```python
from build123d import *

# Parameters (mm, degrees)
SKETCH2_W                       = 27.178
SKETCH2_H                       = 21.59
INITIAL_EXTRUDE_DEPTH           = 6.35
SKETCH3_W                       = 27.178
SKETCH3_H                       = 1.27
INTIAL_EXTRUDE_HORIZONTAL_DEPTH = 12.192
SKETCH4_W                       = 27.178
SKETCH4_H                       = 1.27
SLIGHT_EXTRUDE_VERTICAL_DEPTH   = 0.254
SKETCH5_W                       = 3.048
SKETCH5_H                       = 21.59
CUT_EXTRUDE1_DEPTH              = 2.794
CUT_EXTRUDE2_REACH              = 33.537
SKETCH6_W                       = 1.379153921
SKETCH6_H                       = 12.954
SNAP_START                      = 11.473246079
SNAP_HOOK2_DEPTH                = 0.7366
SNAP_START_2                    = 8.31223189
SNAP_HOOK2_2_DEPTH              = 8.568362063
SNAP_START_3                    = 8.179116131
SNAP_HOOK2_3_DEPTH              = 8.834593581
SNAP_START_4                    = 9
SNAP_HOOK2_4_DEPTH              = 6
BOSS_EXTRUDE1_DEPTH             = 7.54
SKETCH8_W                       = 24.419692158
SKETCH8_H                       = 7.195933706
CUT_EXTRUDE3_DEPTH              = 0.762
SKETCH9_W                       = 24.419692158
SKETCH9_H                       = 20.32
BOSS_EXTRUDE2_DEPTH             = 2.794
SKETCH10_R                      = 5.08
CUT_EXTRUDE4_DEPTH              = 5.08


with BuildPart() as part:
    # Sketch2 → Initial Extrude (new body)
    with BuildSketch(Plane.XY):
        Rectangle(SKETCH2_W, SKETCH2_H)
    extrude(amount=INITIAL_EXTRUDE_DEPTH)

    # Sketch3 → Intial Extrude horizontal (add)
    with BuildSketch(Plane.XY.offset(6.35)):
        with Locations((0, 10.16)):
            Rectangle(SKETCH3_W, SKETCH3_H)
    extrude(amount=INTIAL_EXTRUDE_HORIZONTAL_DEPTH)

    # Sketch4 → Slight Extrude vertical (add)
    with BuildSketch(Plane.XZ.offset(-9.525)):
        with Locations((0, 17.907)):
            Rectangle(SKETCH4_W, SKETCH4_H)
    extrude(amount=SLIGHT_EXTRUDE_VERTICAL_DEPTH)

    # Sketch5 → Cut-Extrude1 (cut)
    with BuildSketch(Plane.ZY.offset(13.589)):
        with Locations((4.064, 0)):
            Rectangle(SKETCH5_W, SKETCH5_H)
    cut_extrude1 = extrude(amount=-CUT_EXTRUDE1_DEPTH, mode=Mode.SUBTRACT)

    # Mirror3: Cut-Extrude1 across plane
    add(cut_extrude1.mirror(Plane(origin=(0, 0, 0), x_dir=(0, 0, 1), z_dir=(1, 0, 0))), mode=Mode.SUBTRACT)

    # Sketch6 → Cut-Extrude2 (cut, up to next)
    with BuildSketch(Plane(origin=(0, 10.795, 0), x_dir=(1, 0, 0), z_dir=(0, 1, 0)), mode=Mode.PRIVATE) as cut_extrude2_sk1:
        with Locations((12.89942304, -12.065)):
            Rectangle(SKETCH6_W, SKETCH6_H)
    cut_extrude2_tool1 = extrude(cut_extrude2_sk1.sketch, amount=-CUT_EXTRUDE2_REACH, mode=Mode.PRIVATE) & part.part
    cut_extrude2 = cut_extrude2_tool1.solids().sort_by_distance((12.899423, 10.795, 12.065))[0]
    add(cut_extrude2, mode=Mode.SUBTRACT)

    # Mirror7: Cut-Extrude2 across plane
    add(cut_extrude2.mirror(Plane(origin=(0, 0, 0), x_dir=(0, 0, 1), z_dir=(1, 0, 0))), mode=Mode.SUBTRACT)

    # Snap Hook2: read off the stored shape, not the designer's step
    # Snap Hook2 outline → Snap Hook2 (add)
    with BuildSketch(Plane.YZ.offset(SNAP_START)):
        Polygon((10.795, 17.013709712), (10.795, 8.179116131), (15.113, 8.405412922), (15.113, 16.787412922), align=None)
    snap_hook2 = extrude(amount=SNAP_HOOK2_DEPTH)

    # Snap Hook2 2 outline → Snap Hook2 2 (add)
    with BuildSketch(Plane.XY.offset(SNAP_START_2)):
        Polygon((11.473246079, 10.795), (11.473246079, 15.113), (10.177846079, 10.795), align=None)
        Polygon((12.209846079, 15.113), (12.209846079, 13.335), (14.241846079, 13.335), (14.241846079, 14.605), align=None)
    snap_hook2_2 = extrude(amount=SNAP_HOOK2_2_DEPTH)

    # Snap Hook2 3 outline → Snap Hook2 3 (add)
    with BuildSketch(Plane.XY.offset(SNAP_START_3)):
        Polygon((11.473246079, 10.795), (11.473246079, 15.113), (10.177846079, 10.795), align=None)
    snap_hook2_3 = extrude(amount=SNAP_HOOK2_3_DEPTH)

    # Snap Hook2 4 outline → Snap Hook2 4 (cut)
    with BuildSketch(Plane.YZ.offset(SNAP_START_4)):
        Polygon((10.795, 8.179116131), (17, 8.179116131), (17, 8.504306402), (15.113, 8.405412922), align=None)
        Polygon((15.113, 16.787412922), (17, 16.688519443), (17, 17.013709712), (10.795, 17.013709712), align=None)
    snap_hook2_4 = extrude(amount=SNAP_HOOK2_4_DEPTH, mode=Mode.SUBTRACT)

    # Mirror6: Snap Hook2, Snap Hook2 2, Snap Hook2 3, Snap Hook2 4 across plane
    add(snap_hook2.mirror(Plane(origin=(0, 0, 0), x_dir=(0, 0, 1), z_dir=(1, 0, 0))))
    add(snap_hook2_2.mirror(Plane(origin=(0, 0, 0), x_dir=(0, 0, 1), z_dir=(1, 0, 0))))
    add(snap_hook2_3.mirror(Plane(origin=(0, 0, 0), x_dir=(0, 0, 1), z_dir=(1, 0, 0))))
    add(snap_hook2_4.mirror(Plane(origin=(0, 0, 0), x_dir=(0, 0, 1), z_dir=(1, 0, 0))), mode=Mode.SUBTRACT)

    # Sketch7 → Boss-Extrude1 (add)
    with BuildSketch(Plane(origin=(0, 10.795, 0), x_dir=(1, 0, 0), z_dir=(0, 1, 0))):
        Polygon((-8.962447439, -8.179116131), (-8.962447439, -18.542), (8.962447439, -18.542), (8.962447439, -8.179116131), (9, -8.179116131), (10.177846079, -8.179116131), (12.209846079, -8.179116131), (12.209846079, -5.588), (10.795, -5.588), (10.795, -2.54), (13.589, -2.54), (13.589, 0), (-13.589, 0), (-13.589, -2.54), (-10.795, -2.54), (-10.795, -5.588), (-12.209846079, -5.588), (-12.209846079, -8.179116131), (-10.177846079, -8.179116131), (-9, -8.179116131), align=None)
    extrude(amount=BOSS_EXTRUDE1_DEPTH)

    # Sketch8 → Cut-Extrude3 (cut)
    with BuildSketch(Plane.XZ.offset(-9.525)):
        with Locations((0, 13.674033147)):
            Rectangle(SKETCH8_W, SKETCH8_H)
    extrude(amount=-CUT_EXTRUDE3_DEPTH, mode=Mode.SUBTRACT)

    # Sketch9 → Boss-Extrude2 (add)
    with BuildSketch(Plane.XY.offset(6.35)):
        with Locations((0, -0.635)):
            Rectangle(SKETCH9_W, SKETCH9_H)
    extrude(amount=BOSS_EXTRUDE2_DEPTH)

    # Sketch10 → Cut-Extrude4 (cut)
    with BuildSketch(Plane(origin=(0, 18.335, 0), x_dir=(1, 0, 0), z_dir=(0, 1, 0))):
        with Locations(Location((0, -12.7, 0), (0, 0, 270))):
            Circle(SKETCH10_R)
    extrude(amount=-CUT_EXTRUDE4_DEPTH, mode=Mode.SUBTRACT)


solid = part.part
```
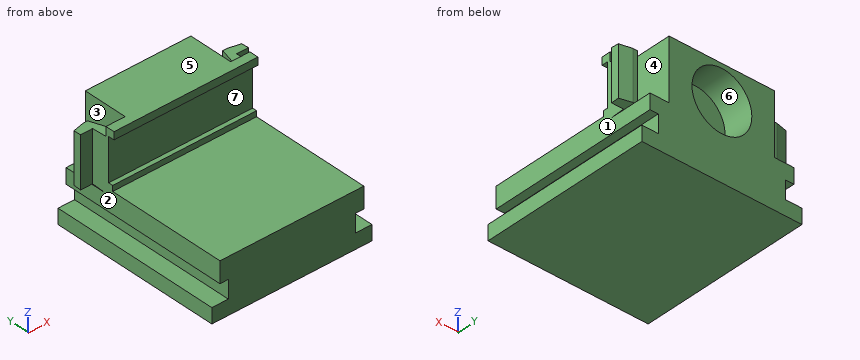
Could you check a few things on this model? Use its own coordinates, in mm. Face numbers are marked on the shaded views. A direction names the side the tool comes from. Coordinates: 2 decimals unless noted, no trailing zeros. Order: outer loops, then holes, each group sorted by start corner. A loop starts at its lowest first (then second) coordinate and runs counter-clockwise, first axis right, second up. Notation, with made-up numbers: M 52.5,-34.5 L 71.5,-34.5 A11 ccw 71.5,-24.5 Z; hole C -37,22 d2. An arc over 180 degrees is marked long. Use one line per item in the form item = value. Start each with the question number.
1. Please list where these lines run through material, in increasing order: line 1 (X direction, y = 16.5, z = 12.7); line 2 (Z direction, x = 9.75, y = 10); line 3 (X direction, y = 14.25, z = 15).
2. Suppose I cut it at C-C on y = -2.5. Write out the boundary of the cut face in (x, z) (3 decimals), then the cut area to 3 significant figures.
3. Suppose I cut it at D-D on z = 16. Write out the boundary of the cut face in (x, y) (3 decimals), then the cut area to 3 significant figures.
4. We'd pull the mould along X, two halves only. Please class the marked faces 1, 2, 3 and 4: +X half, -X half, draft (parallel to the pull), parting line (faces both ways), or undercut.
5. Suppose I cut it at A-A on x = 0. Write out the boundary of the cut face in (y, z) (3 decimals), then the cut area to 3 significant figures.
6. For pin 1 (3 mm diameter, centred on x = 11.5, y = 5.5, fed in from +Z); pin 2 (1 mm diameter, centred on x = 11, y = 15, fed in from +Z); pin 3 (1.5 mm diameter, centred on y = 11, z = 11, fed in from +X), each with a flat end and sliding along its axis, tell me the tip position at first contact or that it passes through.
7. On a 3-axis mill with a long thin cutter (end or side, diameter ignored), from which of +Z, -Z, +X, -X, +Y, -Y can I reach the whole of each face in a straight line? I mean the marked faces 5, 6 and 7. Say none if no direction works.
8. Suppose I cut it at B-B on z = 12.7. Write out the boundary of the cut face in (x, y) (3 decimals).
Geometry says:
q1.line_1 = -8.96 to -5.08, 5.08 to 8.96
q1.line_2 = 0 to 10.08, 17.27 to 18.54
q1.line_3 = -14.24 to -11.21, -8.96 to -4.53, 4.53 to 8.96, 11.21 to 14.24
q2.outline = M -13.589,0 L 13.589,0 L 13.589,2.54 L 10.795,2.54 L 10.795,5.588 L 12.21,5.588 L 12.21,9.144 L -12.21,9.144 L -12.21,5.588 L -10.795,5.588 L -10.795,2.54 L -13.589,2.54 Z
q2.area = 222 mm^2
q3.outline = M -14.242,13.335 L -12.21,13.335 L -12.21,10.287 L 12.21,10.287 L 12.21,13.335 L 14.242,13.335 L 14.242,14.605 L 12.21,15.113 L 11.473,15.113 L 10.178,10.795 L 8.962,10.795 L 8.962,18.335 L 3.862,18.335 L 3.862,13.255 L -3.862,13.255 L -3.862,18.335 L -8.962,18.335 L -8.962,10.795 L -10.178,10.795 L -11.473,15.113 L -12.21,15.113 L -14.242,14.605 Z
q3.area = 126 mm^2
q4.face_1 = +X half
q4.face_2 = -X half
q4.face_3 = undercut
q4.face_4 = undercut
q5.outline = M -10.795,0 L 18.335,0 L 18.335,7.62 L 13.255,7.62 L 13.255,17.78 L 18.335,17.78 L 18.335,18.542 L 9.271,18.542 L 9.271,17.272 L 10.287,17.272 L 10.287,10.076 L 9.525,10.076 L 9.525,9.144 L -10.795,9.144 Z
q5.area = 292 mm^2
q6.pin_1 = 9.14
q6.pin_2 = 16.81
q6.pin_3 = 12.21
q7.face_5 = +Z, +X, -X, +Y, -Y
q7.face_6 = +Y
q7.face_7 = +X, -X, -Y
q8.outline = M -14.242,13.335 L -12.21,13.335 L -12.21,10.287 L 12.21,10.287 L 12.21,13.335 L 14.242,13.335 L 14.242,14.605 L 12.21,15.113 L 11.473,15.113 L 10.178,10.795 L 8.962,10.795 L 8.962,18.335 L 5.08,18.335 L 5.08,13.255 L -5.08,13.255 L -5.08,18.335 L -8.962,18.335 L -8.962,10.795 L -10.178,10.795 L -11.473,15.113 L -12.21,15.113 L -14.242,14.605 Z
